Read the model definition and answer for the solid it produces. Units are mm, in the model's axes. Coordinates: 2 decimals unless noted, no trailing zeros. Loops run counter-clockwise (first coordinate to the right, second up) from the corner with the lowest first, then second, coordinate; pieces in that order, holes last.
Q1. The mould has two halves that part along Y. Classify faces 1 (the face through (-0.325, -15.464, 5.423)), 2 (the face through (-11.99, 0.53, 5.42)), 3 (the face through (8.767, -16.856, 0.578)), 4 (the face through (12, -4, 11)): pulls with the +Y half, pulls with the -Y half, needs draft (parallel to the pull), parting line crosses it, or undercut.
Q2. Section A-A (x = 0) is taken. Give the vertices of the cut face in (y, z).
Q3. Section B-B (z = 8.25) is taken. Give the vertices of the cut face in (x, y).
Q4. Straight lines are drawn through the part: line 1 (X direction, y = 1, z = 1.5); line 2 (X direction, y = -0.5, z = 4); line 3 (Y direction, x = 0, z = 3). For each, find the intervals that lie inside material, in ascending order.
Q5. Section C-C (z = 5.25) is taken. Give the vertices of the cut face in (x, y).
Q6. Flat-ended cylindrical pins translate along their axes: P1, Ø5, axis at y = 10.5, z = 6, coming from the +X side; P2, Ø1.5, axis at y = 6.5, z = 2.5, coming from the -X side; P3, Ø1, axis at y = 8, z = 5, coming from the -X side. Find the tip coordinate at first contact, or state that the pin passes through.
from build123d import *

# Parameters (mm, degrees)
SCHIZZO1_R                   = 19
SCHIZZO1_R_2                 = 12
SCHIZZO1_R_3                 = 1.5
ESTRUSIONE_ESTRUSIONE1_DEPTH = 11
SCHIZZO2_R                   = 3


with BuildPart() as part:
    # Schizzo1 → Estrusione-Estrusione1 (new body)
    with BuildSketch(Plane.XY):
        Circle(SCHIZZO1_R)
        Circle(SCHIZZO1_R_2, mode=Mode.SUBTRACT)
        with Locations((0, 14)):
            Circle(SCHIZZO1_R_3, mode=Mode.SUBTRACT)
        with Locations((14, 0)):
            Circle(SCHIZZO1_R_3, mode=Mode.SUBTRACT)
        with Locations((0, -14)):
            Circle(SCHIZZO1_R_3, mode=Mode.SUBTRACT)
        with Locations((-14, 0)):
            Circle(SCHIZZO1_R_3, mode=Mode.SUBTRACT)
    extrude(amount=ESTRUSIONE_ESTRUSIONE1_DEPTH)

    # Schizzo2 → Taglia-Rivoluzione1 (revolve, cut)
    with BuildSketch(Plane(origin=(0, 0, 0), x_dir=(0, 0, -1), z_dir=(1, 0, 0))):
        with Locations((-4, 20)):
            Circle(SCHIZZO2_R)
    revolve(axis=Axis((0, 0, 11), (0, 0, -1)), mode=Mode.SUBTRACT)


solid = part.part
Numbers:
1. face 1: undercut
1. face 2: undercut
1. face 3: parting line crosses it
1. face 4: needs draft
2. outline: (-19, 0) - (-15.5, 0) - (-15.5, 11) - (-19, 11) - (-19, 6.83) arc R3 cw to (-19, 1.17) - close; (-12.5, 0) - (-12, 0) - (-12, 11) - (-12.5, 11) - close; (12, 0) - (12.5, 0) - (12.5, 11) - (12, 11) - close; (15.5, 0) - (19, 0) - (19, 1.17) arc R3 cw to (19, 6.83) - (19, 11) - (15.5, 11) - close
3. outline: circle Ø38 at (0, 0); hole circle Ø3 at (-14, 0); hole circle Ø24 at (0, 0); hole circle Ø3 at (0, -14); hole circle Ø3 at (0, 14); hole circle Ø3 at (14, 0)
4. line 1: x = -18.31 to -15.12, -12.88 to -11.96, 11.96 to 12.88, 15.12 to 18.31
4. line 2: x = -16.99 to -15.41, -12.59 to -11.99, 11.99 to 12.59, 15.41 to 16.99
4. line 3: y = -17.17 to -15.5, -12.5 to -12, 12 to 12.5, 15.5 to 17.17
5. outline: circle Ø34.55 at (0, 0); hole circle Ø3 at (-14, 0); hole circle Ø24 at (0, 0); hole circle Ø3 at (0, -14); hole circle Ø3 at (0, 14); hole circle Ø3 at (14, 0)
6. P1: stops at x = 17.17
6. P2: stops at x = -16.85
6. P3: stops at x = -15.54
